Verification items for the finished model (mm, model axes). A direction names the side the tool comes from. Coordinates: 2 decimals unless noted, no trailing zeros. Loops run counter-clockwise (first coordinate to the right, second up) from the corner with the lowest first, then second, coordinate; pieces in that order, holes last. Notation, with made-up numbers: (85.5, -13) -> (101.5, -13) arc R30 ccw to (101.5, 9) -> close; hole circle Ø3 at (87, 4.25). An arc over 180 degrees is marked (long way). Use CSV: the item, a comma, the result in double quotes. Start each with the question number.
```python
from build123d import *

# Parameters (mm, degrees)
SKETCH1_W           = 40
SKETCH1_H           = 40
BOSS_EXTRUDE1_DEPTH = 40
SKETCH2_R           = 11
CUT_EXTRUDE1_DEPTH  = 2
SKETCH3_R           = 5
CUT_EXTRUDE2_DEPTH  = 2


with BuildPart() as part:
    # Sketch1 → Boss-Extrude1 (new body)
    with BuildSketch(Plane.XY):
        Rectangle(SKETCH1_W, SKETCH1_H)
    extrude(amount=BOSS_EXTRUDE1_DEPTH)

    # Sketch2 → Cut-Extrude1 (cut)
    with BuildSketch(Plane.XZ.offset(20)):
        with Locations(Location((0, 15, 0), (0, 0, 270))):
            Circle(SKETCH2_R)
    extrude(amount=-CUT_EXTRUDE1_DEPTH, mode=Mode.SUBTRACT)

    # Sketch3 → Cut-Extrude2 (cut)
    with BuildSketch(Plane.XZ.offset(18)):
        with Locations(Location((0, 15, 0), (0, 0, 270))):
            Circle(SKETCH3_R)
    extrude(amount=-CUT_EXTRUDE2_DEPTH, mode=Mode.SUBTRACT)


solid = part.part
```
1. Set-up check for faces 1 (the cylindrical face through (0, -17, 20)), 2 (the flat face through (-20, 0, 20)): record each of +Z, -Z, +X, -X, +Y, -Y from which the full face is reachable in a straight line by a thin tool's end or side.
2. Cross-section at D-D, the plane z = 7.5. Record the boundary of the cut face in (x, y).
3. Cross-section at B-B, the plane x = 0. Record the boundary of the cut face in (y, z).
4. Scan lines: line 1 (X direction, y = -16.75, z = 15); line 2 (X direction, y = -18.6, z = 15); line 3 (Y direction, x = -8, z = 11.5). Record each from-to range of solid material in increasing order.
5. Cross-section at C-C, the plane z = 21. Record the boundary of the cut face in (x, y), plus the area to 3 significant figures.
6. Cross-section at A-A, the plane z = 15. Record the boundary of the cut face in (x, y), plus the area to 3 significant figures.
7. Release check for a two-part mould opening along Z. For faces 3 (the flat face through (0, -16, 15)), 4 (the flat face through (20, 0, 20)), 5 (the flat face through (0, 0, 0)) record: released by +Z, released by -Z, zero draft, split by the parting line, or undercut.
8. Depth check by flat-ended pin: pin 1 (16 mm diameter, centred on x = 0, z = 15, fed in from -Y). Enter the tip coordinate at first touch or a pass-through.
Solution:
1,face 1,"-Y"
1,face 2,"+Z, -Z, -X, +Y, -Y"
2,outline,"(-20, -20) -> (-8.05, -20) -> (-8.05, -18) -> (8.05, -18) -> (8.05, -20) -> (20, -20) -> (20, 20) -> (-20, 20) -> close"
3,outline,"(-20, 0) -> (20, 0) -> (20, 40) -> (-20, 40) -> (-20, 26) -> (-18, 26) -> (-18, 20) -> (-16, 20) -> (-16, 10) -> (-18, 10) -> (-18, 4) -> (-20, 4) -> close"
4,line 1,"x = -20 to -5, 5 to 20"
4,line 2,"x = -20 to -11, 11 to 20"
4,line 3,"y = -18 to 20"
5,outline,"(-20, -20) -> (-9.22, -20) -> (-9.22, -18) -> (9.22, -18) -> (9.22, -20) -> (20, -20) -> (20, 20) -> (-20, 20) -> close"
5,area,"1,560 mm2"
6,outline,"(-20, -20) -> (-11, -20) -> (-11, -18) -> (-5, -18) -> (-5, -16) -> (5, -16) -> (5, -18) -> (11, -18) -> (11, -20) -> (20, -20) -> (20, 20) -> (-20, 20) -> close"
6,area,"1,540 mm2"
7,face 3,"undercut"
7,face 4,"zero draft"
7,face 5,"released by -Z"
8,pin 1,"stops at y = -18"
